Can you work these out from the model? Positions are in its coordinate system, mm. Face numbers are marked on the shaded views. A direction names the side the tool comes from. Give positions to 0.01 mm unless a question says otherwise; leave off trailing zeros. Loops run counter-clockwise (first coordinate to the right, second up) from the corner with the lowest first, then second, coordinate; pieces in that order, holes last.
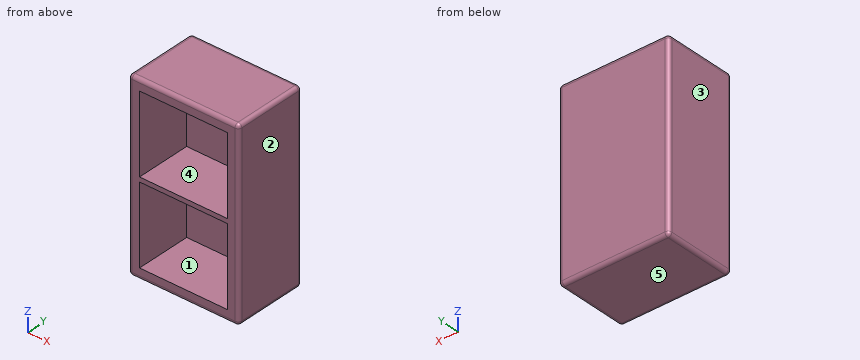
from build123d import *

# Parameters (mm, degrees)
F1_DEPTH = 127
F2_W     = 121.92
F2_H     = 223.52
F3_DEPTH = 76.2
F4_R     = 5.08
F5_W     = 121.92
F5_H     = 6.35
F6_DEPTH = 76.2


with BuildPart() as f1:
    # F0 (on Top) → F1 (new body, symmetric)
    with BuildSketch(Plane.XY):
        Polygon((-76.2, 50.8), (-76.2, -50.8), (-68.293229, -50.8), (68.293229, -50.8), (76.2, -50.8), (76.2, 50.8), align=None)
    extrude(amount=F1_DEPTH, both=True)

    # F2 (on face) → F3 (cut)
    with BuildSketch(Plane.XZ.offset(50.8)):
        Rectangle(F2_W, F2_H)
    extrude(amount=-F3_DEPTH, mode=Mode.SUBTRACT)

    # F4
    f4_edges = [f1.edges().sort_by_distance(p)[0] for p in [
        (76.2, 0, 127),
        (0, -50.8, 127),
        (-76.2, 0, 127),
        (0, 50.8, 127),
        (76.2, -50.8, 0),
        (-76.2, -50.8, 0),
        (76.2, 50.8, 0),
        (76.2, 0, -127),
        (0, -50.8, -127),
        (-76.2, 50.8, 0),
        (0, 50.8, -127),
        (-76.2, 0, -127),
    ]]
    fillet(f4_edges, radius=F4_R)

    # F5 (on face) → F6 (join)
    with BuildSketch(Plane.XZ.offset(-25.4)):
        Rectangle(F5_W, F5_H)
    extrude(amount=F6_DEPTH)


solid = f1.part
(1) Which directions (+Z, -Z, +X, -X, +Y, -Y) give clear straight access to the entire face, cutting with the end or side of a thin tool? Please do the marked faces 4 and 5.
Returned:
face 4: -Y
face 5: -Z, +X, -X, +Y, -Y
(2) Suppose I cut it at B-B on z = 106. List the corners of the cut face in (x, y) for me.
Returned:
outline: (-76.2, -45.72) arc R5.08 ccw to (-71.12, -50.8) - (-60.96, -50.8) - (-60.96, 25.4) - (60.96, 25.4) - (60.96, -50.8) - (71.12, -50.8) arc R5.08 ccw to (76.2, -45.72) - (76.2, 45.72) arc R5.08 ccw to (71.12, 50.8) - (-71.12, 50.8) arc R5.08 ccw to (-76.2, 45.72) - close
(3) Please list where these lines run through material, in increasing order: probe 1 along Z at (x, y) = (-20.5, 24) (3 decimals); probe 2 along X at (y, z) = (9, -49.5); probe 3 along Y at (x, z) = (18.5, 35.5).
Returned:
probe 1: z = -127 to -111.76, -3.175 to 3.175, 111.76 to 127
probe 2: x = -76.2 to -60.96, 60.96 to 76.2
probe 3: y = 25.4 to 50.8
(4) Will this pin go through, and if not, where does the flat tip stop? P1, Ø3, axis at x = -24.5, z = -89, coming from the -Y side.
Returned:
P1: stops at y = 25.4
(5) Thinking about a two-plate mould opening in X: for the marked faces 1, 2 and 3, which applies, pulls with the +X half, pulls with the -X half, needs draft (parallel to the pull), parting line crosses it, or undercut?
Returned:
face 1: undercut
face 2: pulls with the +X half
face 3: pulls with the -X half
(6) Suppose I cut it at C-C on x = 44.5. List the corners of the cut face in (y, z) for me (3 decimals).
Returned:
outline: (-50.8, -121.92) arc R5.08 ccw to (-45.72, -127) - (45.72, -127) arc R5.08 ccw to (50.8, -121.92) - (50.8, 121.92) arc R5.08 ccw to (45.72, 127) - (-45.72, 127) arc R5.08 ccw to (-50.8, 121.92) - (-50.8, 111.76) - (25.4, 111.76) - (25.4, 3.175) - (-50.8, 3.175) - (-50.8, -3.175) - (25.4, -3.175) - (25.4, -111.76) - (-50.8, -111.76) - close
(7) Suppose I cut it at A-A on y = 7. List the corners of the cut face in (x, z) for me (3 decimals).
Returned:
outline: (-76.2, -121.92) arc R5.08 ccw to (-71.12, -127) - (71.12, -127) arc R5.08 ccw to (76.2, -121.92) - (76.2, 121.92) arc R5.08 ccw to (71.12, 127) - (-71.12, 127) arc R5.08 ccw to (-76.2, 121.92) - close; hole (-60.96, -111.76) - (60.96, -111.76) - (60.96, -3.175) - (-60.96, -3.175) - close; hole (-60.96, 3.175) - (60.96, 3.175) - (60.96, 111.76) - (-60.96, 111.76) - close
